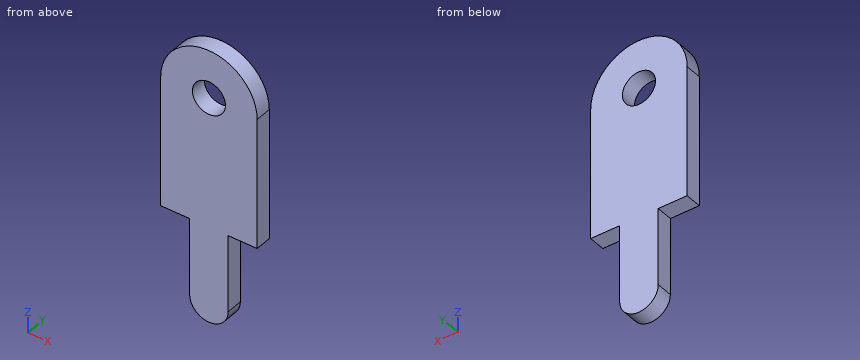
from build123d import *

# Parameters (mm, degrees)
SKETCH_R  = 0.6
PAD_DEPTH = 0.3


with BuildPart() as part:
    # Sketch → Pad (new body, symmetric)
    with BuildSketch(Plane(origin=(0, 0, 0), x_dir=(-1, 0, 0), z_dir=(0, 1, 0))):
        with BuildLine():
            Line((-1.75, 4.75), (-1.75, 0))
            Line((-1.75, 0), (-0.7, 0))
            Line((-0.7, 0), (-0.7, -2.8))
            ThreePointArc((-0.7, -2.8), (0, -3.5), (0.7, -2.8))
            Line((0.7, 0), (0.7, -2.8))
            Line((0.7, 0), (1.75, 0))
            Line((1.75, 0), (1.75, 4.75))
            ThreePointArc((1.75, 4.75), (0, 6.5), (-1.75, 4.75))
        make_face()
        with Locations((0, 4.75)):
            Circle(SKETCH_R, mode=Mode.SUBTRACT)
    extrude(amount=PAD_DEPTH, both=True)


solid = part.part
The listing builds one solid part. Answer for the finished solid, in the listing's coordinates (mm). Round coordinates to 2 decimals unless told otherwise and drop trailing zeros. Order: outer loops, then holes, each group sorted by start corner. A loop starts at its lowest first (then second) coordinate and runs counter-clockwise, first axis right, second up. Notation, with made-up numbers: M 88,86 L 112,86 A24 cw 112,117 Z; hole C 17.5,9.5 d8. An arc over 180 degrees is marked long. Answer in a Markdown table with one row per item. Add a question column.
1) The part is cut by section D-D on z = -1. Determine the outline of the cut face in (x, y), plus the area to 3 significant figures.
2) The part is cut by section A-A on x = 0. Determine the outline of the cut face in (y, z).
3) Consider line 1 along Z through (x, y) = (0, 0.1); line 2 along X through (y, z) = (0.05, 4.25); line 3 along X through (y, z) = (0.1, 4.5). Determine where each line is inside the solid, lowest interval first. Write a range as from..to.
4) The part is cut by section B-B on y = -0.1. Determine the outline of the cut face in (x, z).
5) The part is cut by section C-C on x = 0.45. Determine the outline of the cut face in (y, z), plus the area to 3 significant figures.
Findings below:
| question | item | result |
|---|---|---|
| 1 | outline | M -0.7,-0.3 L 0.7,-0.3 L 0.7,0.3 L -0.7,0.3 Z |
| 1 | area | 0.840 mm² |
| 2 | outline | M -0.3,-3.5 L 0.3,-3.5 L 0.3,4.15 L -0.3,4.15 Z; M -0.3,5.35 L 0.3,5.35 L 0.3,6.5 L -0.3,6.5 Z |
| 3 | line 1 | z = -3.5..4.15, 5.35..6.5 |
| 3 | line 2 | x = -1.75..-0.33, 0.33..1.75 |
| 3 | line 3 | x = -1.75..-0.55, 0.55..1.75 |
| 4 | outline | M -1.75,0 L -0.7,0 L -0.7,-2.8 A0.7 ccw 0.7,-2.8 L 0.7,0 L 1.75,0 L 1.75,4.75 A1.75 ccw -1.75,4.75 Z; hole C 0,4.75 d1.2 |
| 5 | outline | M -0.3,-3.34 L 0.3,-3.34 L 0.3,4.35 L -0.3,4.35 Z; M -0.3,5.15 L 0.3,5.15 L 0.3,6.44 L -0.3,6.44 Z |
| 5 | area | 5.39 mm² |
